Here's how the part is built. I have some questions about the finished solid (model axes, mm). A direction names the side the tool comes from. Give positions to 0.01 mm unless a question says otherwise; leave off trailing zeros. Answer as CSV lines item,"result". Start each with the question number.
Q1. On a 3-axis mill with a long thin cutter (end or side, diameter ignored), from which of +Z, -Z, +X, -X, +Y, -Y can I reach the whole of each face in a straight line? I mean faces 1 (the cylindrical face through (-1.485, 27.097, 29.442)), 2 (the cylindrical face through (6.12, -33.5, 27.62)). Say none if no direction works.
Q2. If I drill on line 1 along Y through (x, z) = (-6.15, 0); line 2 along Z through (x, y) = (-0.75, -1); line 3 along Y through (x, z) = (-3.75, -16.5), over which ranges is the centre line in solid material (lowest first)?
Q3. For pin 1 (6 mm diameter, centred on x = 4.5, y = -22.5, fed in from -Z); pin 2 (4 mm diameter, centred on x = 2, y = -31.5, fed in from +Z); pin 3 (2 mm diameter, centred on x = -1, y = -3, fed in from +Z), each with a flat end and sliding along its axis, tell me the tip position at first contact or that it passes through.
Q4. Suppose I cut it at A-A (z = 0). Count the separate pieces of the cut face and the enclosed holes in it, then the cut area to 3 significant figures.
Q5. Thinking about a two-plate mould opening in Z: for faces 3 (the flat face through (7.5, -11, 32)), 4 (the conical face through (-3.6, 12.69, 30.62)), 5 (the cylindrical face through (-0.1, 46.37, -10.3)), which applies, +Z half, -Z half, draft (parallel to the pull), parting line (faces both ways), or undercut?
```python
from build123d import *

# Parameters (mm, degrees)
FILLET1_R                                    = 2
FILLET2_R                                    = 0.5
CBORE_FOR_M4_HEX_HEAD_CAP_SCREW1_D           = 4.5
CBORE_FOR_M4_HEX_HEAD_CAP_SCREW1_CBORE_D     = 9
CBORE_FOR_M4_HEX_HEAD_CAP_SCREW1_CBORE_DEPTH = 2.8
CIRPATTERN1_COUNT                            = 8


with BuildPart() as part:
    # Sketch1 → Revolve1 (revolve)
    with BuildSketch(Plane.XY, mode=Mode.PRIVATE) as revolve1_sk:
        Polygon((-3.742640687, 33), (0, 36.742640687), (3.742640687, 33), (7.5, 33), (7.5, 47.5), (-7.5, 47.5), (-7.5, 33), align=None)
    revolve(revolve1_sk.sketch.rotate(Axis((-33.732241936, 0, 0), (1, 0, 0)), 90), axis=Axis((-33.732241936, 0, 0), (1, 0, 0)))

    # Fillet1
    fillet1_edges = [part.edges().sort_by_distance(p)[0] for p in [
        (0, 0, -36.742640687),
    ]]
    fillet(fillet1_edges, radius=FILLET1_R)

    # Fillet2
    fillet2_edges = [part.edges().sort_by_distance(p)[0] for p in [
        (-7.5, 0, -47.5),
        (7.5, 0, -47.5),
    ]]
    fillet(fillet2_edges, radius=FILLET2_R)

    # CBORE for M4 Hex Head Cap Screw1 (through all)
    with Locations(Plane(origin=(7.5, 41.5, 0), x_dir=(0, 0, 1), z_dir=(1, 0, 0))):
        with Locations((0, 0)):
            cbore_for_m4_hex_head_cap_screw1 = CounterBoreHole(CBORE_FOR_M4_HEX_HEAD_CAP_SCREW1_D / 2, CBORE_FOR_M4_HEX_HEAD_CAP_SCREW1_CBORE_D / 2, CBORE_FOR_M4_HEX_HEAD_CAP_SCREW1_CBORE_DEPTH)

    # CirPattern1: CBORE for M4 Hex Head Cap Screw1 ×8 about axis
    cirpattern1_axis = Axis((0, 0, 0), (1, 0, 0))
    for i in range(1, CIRPATTERN1_COUNT):
        add(cbore_for_m4_hex_head_cap_screw1.rotate(cirpattern1_axis, i * 360 / CIRPATTERN1_COUNT), mode=Mode.SUBTRACT)


solid = part.part
```
Resolved:
1,face 1,"+X, -X"
1,face 2,"+X"
2,line 1,"-47.5 to -43.75, -39.25 to -33, 33 to 39.25, 43.75 to 47.5"
2,line 2,"-47.49 to -43.52, -39.48 to -35.75, 35.75 to 39.48, 43.52 to 47.49"
2,line 3,"-44.54 to -28.58, 28.58 to 44.54"
3,pin 1,"z = -43.31"
3,pin 2,"z = 37.23"
3,pin 3,"z = 47.46"
4,separate pieces,"4"
4,enclosed holes,"0"
4,area,"248 mm^2"
5,face 3,"draft"
5,face 4,"undercut"
5,face 5,"parting line"
